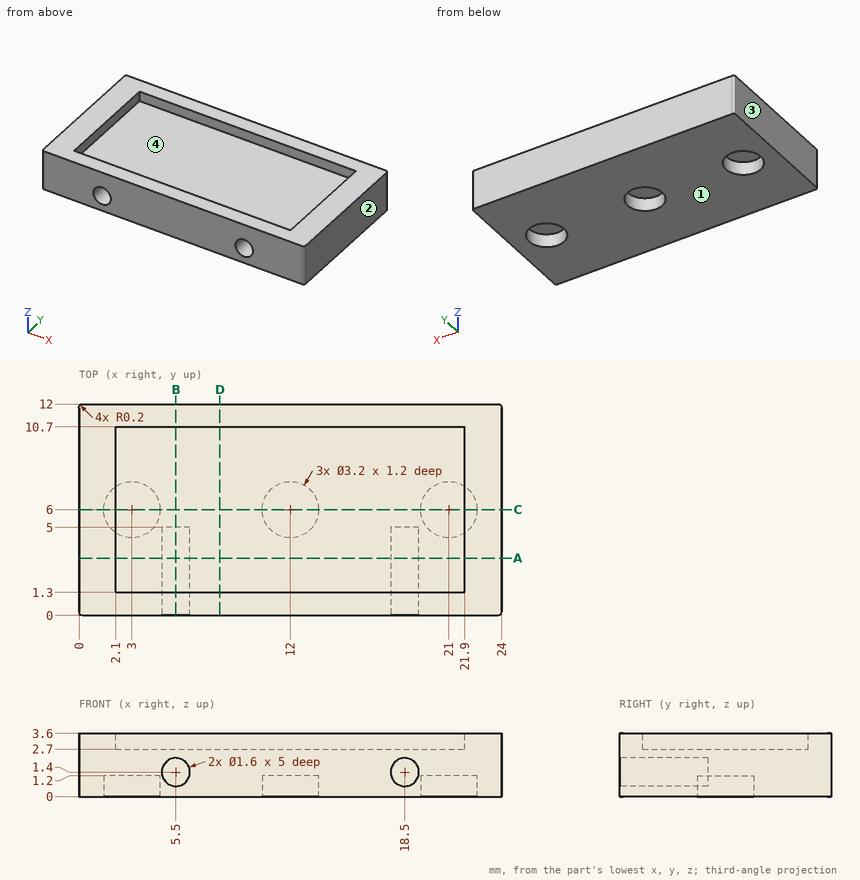
Verification items for this drawing (mm, ordinates from the low corner). Coordinates: 2 decimals unless noted, no trailing zeros. Write each loop counter-clockwise with the first axis right and the second up, starting at its lowest first coordinate (ties: lowest second). Pieces come first, ordered by that corner, then holes. Notation, with made-up numbers: M 32.25,-0.75 L 48.25,-0.75 A29 cw 48.25,34.25 Z; hole C 19.5,-8.5 d11. An arc over 180 degrees is marked long. Answer as a JSON object with one key per item and string values. Group by question number.
(1) Material ranges on line 1 (Y direction, x = 21, z = 0.5); line 2 (X direction, y = 6, z = 0.7); line 3 (X direction, y = 4.5, z = 2.9), recorded low to high.
(2) Cross-section at C-C, the plane y = 6. Record the cut outline in (x, z).
(3) Cross-section at B-B, the plane x = 5.5. Record the cut outline in (y, z).
(4) Cross-section at A-A, the plane y = 3.25. Record the cut outline in (x, z).
(5) Release check for a two-part mould opening along X. For the marked faces 1, 2, 3 and 4 record: +X half, -X half, draft (parallel to the pull), parting line (faces both ways), or undercut.
(6) Cross-section at D-D, the plane x = 8. Record the cut outline in (y, z).
(7) Gauge pin test, flat ends, axial feed: pin 1 (4 mm diameter, centred on x = 15.5, y = 6, fed in from +Z); pin 2 (1.6 mm diameter, centred on x = 12, y = 5.5, fed in from -Z); pin 3 (1.4 mm diameter, centred on x = 5.5, z = 1.4, fed in from -Y). Record the tip position at first contact, or that the pin passes through.
Reply:
{
 "1": {"line 1": "0 to 4.4, 7.6 to 12", "line 2": "0 to 1.4, 4.6 to 10.4, 13.6 to 19.4, 22.6 to 24", "line 3": "0 to 2.1, 21.9 to 24"},
 "2": {"outline": "M 0,0 L 1.4,0 L 1.4,1.2 L 4.6,1.2 L 4.6,0 L 10.4,0 L 10.4,1.2 L 13.6,1.2 L 13.6,0 L 19.4,0 L 19.4,1.2 L 22.6,1.2 L 22.6,0 L 24,0 L 24,3.6 L 21.9,3.6 L 21.9,2.7 L 2.1,2.7 L 2.1,3.6 L 0,3.6 Z"},
 "3": {"outline": "M 0,0 L 12,0 L 12,3.6 L 10.7,3.6 L 10.7,2.7 L 1.3,2.7 L 1.3,3.6 L 0,3.6 L 0,2.2 L 5,2.2 L 5,0.6 L 0,0.6 Z"},
 "4": {"outline": "M 0,0 L 24,0 L 24,3.6 L 21.9,3.6 L 21.9,2.7 L 2.1,2.7 L 2.1,3.6 L 0,3.6 Z; hole C 5.5,1.4 d1.6; hole C 18.5,1.4 d1.6"},
 "5": {"face 1": "draft", "face 2": "+X half", "face 3": "-X half", "face 4": "undercut"},
 "6": {"outline": "M 0,0 L 12,0 L 12,3.6 L 10.7,3.6 L 10.7,2.7 L 1.3,2.7 L 1.3,3.6 L 0,3.6 Z"},
 "7": {"pin 1": "z = 2.7", "pin 2": "z = 1.2", "pin 3": "y = 5"}
}
